Build history of the part. All positions in model axes, mm. A direction names the side the tool comes from. Round coordinates to 2 decimals unless told otherwise and drop trailing zeros. Write each loop counter-clockwise with the first axis right and the second up, starting at its lowest first coordinate (ties: lowest second). Pieces come first, ordered by that corner, then holes. Notation, with made-up numbers: (-8, 84) -> (4, 84) arc R6 cw to (4, 89) -> close; hole circle Ø4 at (-38, -6). An arc over 180 degrees is marked (long way). Answer in a Markdown table with one row per item.
```python
from build123d import *

# Parameters (mm, degrees)
F2_W          = 44
F2_H          = 44
F2_R          = 15
F2_R_2        = 10
F3_DEPTH      = 60
F4_R          = 15
F4_R_2        = 10
F5_DEPTH      = 7
F6_DEPTH      = 9
F8_SIZE       = 2
F11_DEPTH     = 60
F12_T4_ANGLE  = 332.4696617
F12_T9_ANGLE  = 152.2075678766
F12_T14_ANGLE = 152.2075678766
F12_T19_ANGLE = 332.4696617


# Not quite as in the source:
# - a fillet or chamfer that OpenCascade refuses, or shapes differently, is made with other operations: its cross-section is extruded or revolved along the edge and cut away or added


with BuildPart() as f3:
    # F2 (on Top) → F3 (new body)
    with BuildSketch(Plane.XY):
        Rectangle(F2_W, F2_H)
        Circle(F2_R, mode=Mode.SUBTRACT)
        Circle(F2_R)
        Circle(F2_R_2, mode=Mode.SUBTRACT)
        Circle(F2_R_2)
    extrude(amount=F3_DEPTH)

    # F4 (on face) → F5 (join)
    with BuildSketch(Plane.XY.offset(60)):
        Circle(F4_R)
        Circle(F4_R_2, mode=Mode.SUBTRACT)
        Circle(F4_R_2)
    extrude(amount=F5_DEPTH)

    # F2 (on Top) → F6 (cut)
    with BuildSketch(Plane.XY):
        Circle(F2_R)
        Circle(F2_R_2, mode=Mode.SUBTRACT)
        Circle(F2_R_2)
    extrude(amount=F6_DEPTH, mode=Mode.SUBTRACT)

    # F8
    f8_edges = [f3.edges().sort_by_distance(p)[0] for p in [
        (0, -22, 0),
        (22, 0, 0),
        (-22, 0, 0),
        (0, 22, 0),
        (-22, -22, 30),
        (-22, 22, 30),
        (22, 22, 30),
        (22, -22, 30),
        (22, 0, 60),
        (0, -22, 60),
        (-22, 0, 60),
        (0, 22, 60),
        (-15, 0, 0),
    ]]
    chamfer(f8_edges, length=F8_SIZE)

    # F10 (on offset) → F11 (cut)
    with BuildSketch(Plane.YZ.offset(22)):
        with BuildLine():
            ThreePointArc((10, 52.5087859035), (7.0710678119, 59.5798537153), (0, 62.5087859035))
            Line((0, 62.5087859035), (0, 42.5087859035))
            ThreePointArc((0, 42.5087859035), (7.0710678119, 45.4377180916), (10, 52.5087859035))
        make_face()
        with BuildLine():
            Line((0, 42.5087859035), (0, 62.5087859035))
            ThreePointArc((0, 62.5087859035), (-10, 52.5087859035), (0, 42.5087859035))
        make_face()
    extrude(amount=-F11_DEPTH, mode=Mode.SUBTRACT)

    # F12: chamfer of 3 x 8 on 4 edges, made by hand


with BuildPart() as f12_tool2:
    # F12_s3 → F12_t4 (revolve)
    with BuildSketch(Plane(origin=(0, -21.5222750688, 41.2905103072), x_dir=(1, 0, 0), z_dir=(0, 0.4622182236, -0.8867662115))):
        Polygon((-22, -37.2705177426), (-14, -34.2705177426), (-22, -34.2705177426), align=None)
    revolve(axis=Axis((-22, 0, 52.5087859035), (1, 0, 0)), revolution_arc=F12_T4_ANGLE)

    split(bisect_by=Plane.XY.offset(60), keep=Keep.BOTTOM)


with BuildPart() as f3_1:
    add(f3.part)

    # F12_t1: cut F12_tool2
    add(f12_tool2.part, mode=Mode.SUBTRACT)


with BuildPart() as f12_tool7:
    # F12_s8 → F12_t9 (revolve)
    with BuildSketch(Plane.XY.offset(52.5087859035)):
        Polygon((-22, 13), (-14, 10), (-22, 10), align=None)
    revolve(axis=Axis((-22, 0, 52.5087859035), (1, 0, 0)), revolution_arc=F12_T9_ANGLE)

    split(bisect_by=Plane.XY.offset(60), keep=Keep.BOTTOM)


with BuildPart() as f3_2:
    add(f3_1.part)

    # F12_t6: cut F12_tool7
    add(f12_tool7.part, mode=Mode.SUBTRACT)


with BuildPart() as f12_tool12:
    # F12_s13 → F12_t14 (revolve)
    with BuildSketch(Plane.XY.offset(52.5087859035)):
        Polygon((22, 13), (14, 10), (22, 10), align=None)
    revolve(axis=Axis((22, 0, 52.5087859035), (1, 0, 0)), revolution_arc=F12_T14_ANGLE)

    split(bisect_by=Plane.XY.offset(60), keep=Keep.BOTTOM)


with BuildPart() as f3_3:
    add(f3_2.part)

    # F12_t11: cut F12_tool12
    add(f12_tool12.part, mode=Mode.SUBTRACT)


with BuildPart() as f12_tool17:
    # F12_s18 → F12_t19 (revolve)
    with BuildSketch(Plane(origin=(0, -21.5222750688, 41.2905103072), x_dir=(1, 0, 0), z_dir=(0, 0.4622182236, -0.8867662115))):
        Polygon((22, -37.2705177426), (14, -34.2705177426), (22, -34.2705177426), align=None)
    revolve(axis=Axis((22, 0, 52.5087859035), (1, 0, 0)), revolution_arc=F12_T19_ANGLE)

    split(bisect_by=Plane.XY.offset(60), keep=Keep.BOTTOM)


with BuildPart() as f3_4:
    add(f3_3.part)

    # F12_t16: cut F12_tool17
    add(f12_tool17.part, mode=Mode.SUBTRACT)


solid = f3_4.part
```
Q1. Saw through at B-B on y = 18. Write the cut outline in (x, z), plus the area to 3 significant figures.
A:
| item | result |
|---|---|
| outline | (-22, 2) -> (-20, 0) -> (20, 0) -> (22, 2) -> (22, 58) -> (20, 60) -> (-20, 60) -> (-22, 58) -> close |
| area | 2,630 mm² |
Q2. Saw through at C-C on z = 61.5. Write the cut outline in (x, y).
A:
| item | result |
|---|---|
| outline | (-14.35, -4.38) arc R15 ccw to (14.35, -4.38) -> close; (-14.35, 4.38) -> (14.35, 4.38) arc R15 ccw to start |
Q3. Wall check: line 1 (Y direction, x = 0, z = 5); line 2 (Z direction, x = 3.5, y = -18); line 3 (X direction, y = 11.5, z = 5). Give the ranges that are in metal, low to high. Write a range as [from, to].
A:
| item | result |
|---|---|
| line 1 | [-22, -15], [15, 22] |
| line 2 | [0, 60] |
| line 3 | [-22, -9.63], [9.63, 22] |
Q4. Two-plate mould, pull along X, no slides. Class faces 1 (the flat face through (-21, -21, 30)), 2 (the cylindrical face through (6.92, -13.31, 63.45)), 3 (the cylindrical face through (-14.985, 0.66, 5.451)): released by +X, released by -X, zero draft, split by the parting line, or undercut.
A:
| item | result |
|---|---|
| face 1 | released by -X |
| face 2 | split by the parting line |
| face 3 | undercut |
Q5. Saw through at A-A on x = 0. Write the cut outline in (y, z).
A:
| item | result |
|---|---|
| outline | (-22, 2) -> (-20, 0) -> (-17, 0) -> (-15, 2) -> (-15, 9) -> (15, 9) -> (15, 2) -> (17, 0) -> (20, 0) -> (22, 2) -> (22, 58) -> (20, 60) -> (15, 60) -> (15, 67) -> (-15, 67) -> (-15, 60) -> (-20, 60) -> (-22, 58) -> close; hole circle Ø20 at (0, 52.51) |
Q6. Which spindle directions (+Z, -Z, +X, -X, +Y, -Y) get a long thin tool onto all of the face, cutting with end or side? Do faces 4 (the flat face through (0, 0, 9)), 5 (the flat face through (-21, -15, 59)), 6 (the flat face through (0, 16, 60)), 7 (the flat face through (21, 15, 59)), 8 (the flat face through (0, -16, 60)). Say none if no direction does.
A:
| item | result |
|---|---|
| face 4 | -Z |
| face 5 | +Z, -X, +Y, -Y |
| face 6 | +Z, +Y |
| face 7 | +Z, +X, +Y, -Y |
| face 8 | +Z, -Y |
Q7. Drop flat-ended pins along their axis: P1, Ø15, axis at x = -5, y = 2.5, coming from the -Z side; P2, Ø1, axis at x = -15.5, y = -11, coming from the +Z side; P3, Ø5, axis at y = 6.5, z = 55.5, coming from the +X side. Give the stop position or say it passes through.
A:
| item | result |
|---|---|
| P1 | z = 9 |
| P2 | z = 60 |
| P3 | through |
